Input: part model. Units: mm. Frame: model coordinates. A direction names the side the tool comes from. Coordinates: 2 decimals unless noted, no trailing zeros. Loops run counter-clockwise (first coordinate to the right, second up) from the corner with the lowest first, then second, coordinate; pieces in that order, holes last. Notation, with made-up numbers: M 3.25,-25 L 15.25,-25 A25 cw 15.25,0 Z; hole C 22,30 d5. An arc over 180 degrees is marked long. Use a Markdown table: item, result. Add a question column.
1. Section A-A on y = 3. Output: boundary loops of the cut face in (x, z).
2. Draft query along X for faces 4 (the flat face through (-30, 47, 0)), 5 (the flat face through (1, 31, -18)), 6 (the cylindrical face through (-50.495, -0.149, -0.242)). Return one class per face: +X half, -X half, draft (parallel to the pull), parting line (faces both ways), or undercut.
3. Section B-B on y = 52.5. Output: boundary loops of the cut face in (x, z).
4. Line query: L1, parallel to Z at x = -45, y = -3.25; L2, parallel to X at y = 52, z = 3; L3, parallel to Y at x = -10.5, z = -7. Output: solid intervals per line, ascending. Write a range as [from, to].
5. Section C-C on z = 8. Output: boundary loops of the cut face in (x, y), then the cut area to 3 significant figures.
6. Section D-D on x = -4.5. State how many separate pieces and enclosed holes the cut face has, then the cut area to 3 significant figures.
7. Pin query (flat end, axial travel): pin 1 (5 mm diameter, centred on y = 34, z = -8.5, fed in from +X); pin 2 (21 mm diameter, centred on x = 49.5, z = 5.5, fed in from +Y); pin 3 (5 mm diameter, centred on y = 83, z = -2.5, fed in from -X); pin 4 (14.5 mm diameter, centred on x = 45, z = 0, fed in from -Y). Return the tip coordinate at first contact, or that it passes through.
8. Set-up query: faces 1 (the flat face through (40, 7.5, 4)), 2 (the flat face through (1, 82.2, 4.3)), 3 (the flat face through (1, 31, 18)). Return all of +Z, -Z, +X, -X, +Y, -Y with unobstructed straight access to the full face (end or side cutting, diameter ignored); none if empty.
```python
from build123d import *

# Parameters (mm, degrees)
BOSS_EXTRUDE1_DEPTH     = 18
SKETCH2_R               = 5.5
CUT_EXTRUDE1_DEPTH      = 101.667770413
CUT_EXTRUDE2_DEPTH      = 108.332427532
CUT_EXTRUDE2_DEPTH_BACK = 108.332427532
SKETCH5_R               = 4.5
CHAMFER2_SIZE           = 0.5
FILLET2_R               = 0.5


with BuildPart() as part:
    # Sketch1 → Boss-Extrude1 (new, symmetric)
    with BuildSketch(Plane.XY):
        with BuildLine():
            Line((-57, -7.5), (-57, 7.5))
            Line((-57, 7.5), (-30, 7.5))
            Line((-30, 7.5), (-30, 88.5))
            Line((-30, 88.5), (-1, 88.5))
            Line((-1, 88.5), (-1, 72.474984355))
            ThreePointArc((-1, 72.474984355), (0, 32.5), (1, 72.474984355))
            Line((1, 72.474984355), (1, 88.5))
            Line((1, 88.5), (30, 88.5))
            Line((30, 88.5), (30, 7.5))
            Line((30, 7.5), (57, 7.5))
            Line((57, 7.5), (57, -7.5))
            Line((57, -7.5), (-57, -7.5))
        make_face()
    extrude(amount=BOSS_EXTRUDE1_DEPTH, both=True)

    # Sketch2 → Cut-Extrude1 (cut, through all)
    with BuildSketch(Plane(origin=(0, 7.5, 0), x_dir=(1, 0, 0), z_dir=(0, 1, 0))):
        with Locations(Location((45, 0, 0), (0, 0, 180))):
            Circle(SKETCH2_R)
        with Locations((-45, 0)):
            Circle(SKETCH2_R)
    extrude(amount=-CUT_EXTRUDE1_DEPTH, mode=Mode.SUBTRACT)

    # Sketch5 → Cut-Extrude2 (cut, two sides: drawn at the far end of the back side and taken through both)
    with BuildSketch(Plane(origin=(-1, 0, 0), x_dir=(0, 0, -1), z_dir=(1, 0, 0)).offset(-CUT_EXTRUDE2_DEPTH_BACK)):
        with Locations((0.330734984, 80.487492178)):
            Circle(SKETCH5_R)
    extrude(amount=CUT_EXTRUDE2_DEPTH + CUT_EXTRUDE2_DEPTH_BACK, mode=Mode.SUBTRACT)

    # Chamfer2
    chamfer2_edges = [part.edges().sort_by_distance(p)[0] for p in [
        (0, 32.5, -18),
        (0, 32.5, 18),
        (50.5, 7.5, 0),
        (-50.5, 7.5, 0),
        (-30, 80.487492178, 4.169265016),
        (30, 80.487492178, 4.169265016),
    ]]
    chamfer(chamfer2_edges, length=CHAMFER2_SIZE)

    # Fillet2
    fillet2_edges = [part.edges().sort_by_distance(p)[0] for p in [
        (-43.5, 7.5, 18),
        (30, 48, -18),
        (43.5, 7.5, -18),
        (-57, 0, 18),
        (57, 0, -18),
        (-57, 0, -18),
        (-43.5, 7.5, -18),
        (-30, 48, -18),
        (57, 0, 18),
        (30, 88.5, 0),
        (57, 7.5, 0),
        (57, -7.5, 0),
        (-57, -7.5, 0),
        (-57, 7.5, 0),
        (-30, 88.5, 0),
        (43.5, 7.5, 18),
        (30, 48, 18),
        (-30, 48, 18),
    ]]
    fillet(fillet2_edges, radius=FILLET2_R)


solid = part.part
```
Answers below:
| question | item | result |
|---|---|---|
| 1 | outline | M -57,-17.5 A0.5 ccw -56.5,-18 L 56.5,-18 A0.5 ccw 57,-17.5 L 57,17.5 A0.5 ccw 56.5,18 L -56.5,18 A0.5 ccw -57,17.5 Z; hole C -45,0 d11; hole C 45,0 d11 |
| 2 | face 4 | -X half |
| 2 | face 5 | draft |
| 2 | face 6 | undercut |
| 3 | outline | M -30,-17.5 A0.5 ccw -29.5,-18 L -20.5,-18 L -20,-17.5 L -20,17.5 L -20.5,18 L -29.5,18 A0.5 ccw -30,17.5 Z; M 20,-17.5 L 20.5,-18 L 29.5,-18 A0.5 ccw 30,-17.5 L 30,17.5 A0.5 ccw 29.5,18 L 20.5,18 L 20,17.5 Z |
| 4 | L1 | z = [-18, -5.5], [5.5, 18] |
| 4 | L2 | x = [-30, -19.99], [19.99, 30] |
| 4 | L3 | y = [-7.5, 35.48], [69.52, 88.5] |
| 5 | outline | M -57,-7 A0.5 ccw -56.5,-7.5 L 56.5,-7.5 A0.5 ccw 57,-7 L 57,7 A0.5 ccw 56.5,7.5 L 30,7.5 L 30,88 A0.5 ccw 29.5,88.5 L 1,88.5 L 1,72.47 A20 cw long -1,72.47 L -1,88.5 L -29.5,88.5 A0.5 ccw -30,88 L -30,7.5 L -56.5,7.5 A0.5 ccw -57,7 Z |
| 5 | area | 5,280 mm² |
| 6 | separate pieces | 2 |
| 6 | enclosed holes | 1 |
| 6 | area | 1,990 mm² |
| 7 | pin 1 | stops at x = 30 |
| 7 | pin 2 | stops at y = 7.5 |
| 7 | pin 3 | stops at x = -30 |
| 7 | pin 4 | stops at y = -7.5 |
| 8 | face 1 | +Z, -Z, +X, +Y |
| 8 | face 2 | +Z, -Z, +Y |
| 8 | face 3 | +Z, +X, -X, +Y, -Y |
